Check sheet for the drawn part. Datum: minimum x, y, z corner. Units: mm. A direction names the side the tool comes from. Give positions to 0.01 mm unless a question says otherwise; leave off trailing zeros. Write each loop counter-clockwise with the first axis right and the second up, starting at its lowest first coordinate (ties: lowest second). Pieces come first, ordered by that corner, then holes. Notation, with made-up numbers: (17.5, -9) -> (36.5, -9) arc R32 cw to (36.5, 25) -> close; hole circle Ø9 at (-39.75, 36). An arc over 180 degrees is marked (long way). Answer as CSV lines item,"result". Start each with the question number.
1) Material ranges on L1, parallel to Y at x = 19, z = 31; L2, parallel to Y at x = 103.5, z = 36.5; L3, parallel to Y at x = 133.35, z = 18, recorded low to high.
2) Sectioned sample at B-B on y = 19.05. Record the cut outline in (x, z).
3) Sectioned sample at C-C on x = 133.35. Record the cut outline in (y, z) (3 decimals).
4) Sectioned sample at A-A on y = 44.5. Record the cut outline in (x, z), and give its area (3 significant figures).
5) Mould release check, pull along Z, two halves, no side actions. Record for the marked faces 4, 5, 6 and 7: released by +Z, released by -Z, zero draft, split by the parting line, or undercut.
6) Sectioned sample at D-D on z = 92. Record the cut outline in (x, y).
7) Gauge pin test, flat ends, axial feed: pin 1 Ø12 at (x, y) = (78, 94) entering from -Z; pin 2 Ø12 at (x, y) = (132.5, 86) entering from -Z; pin 3 Ø14.5 at (x, y) = (133.35, 19.05) entering from +Z; pin 4 Ø10 at (x, y) = (19.05, 19.05) entering from -Z. Record the tip position at first contact, or that the pin passes through.
8) Tool access check on the marked faces 1, 2 and 3. Record the directions out of +Z, -Z, +X, -X, +Y, -Y that give a thin tool (end or side, any length) a straight path to the whole face; none if there is none.
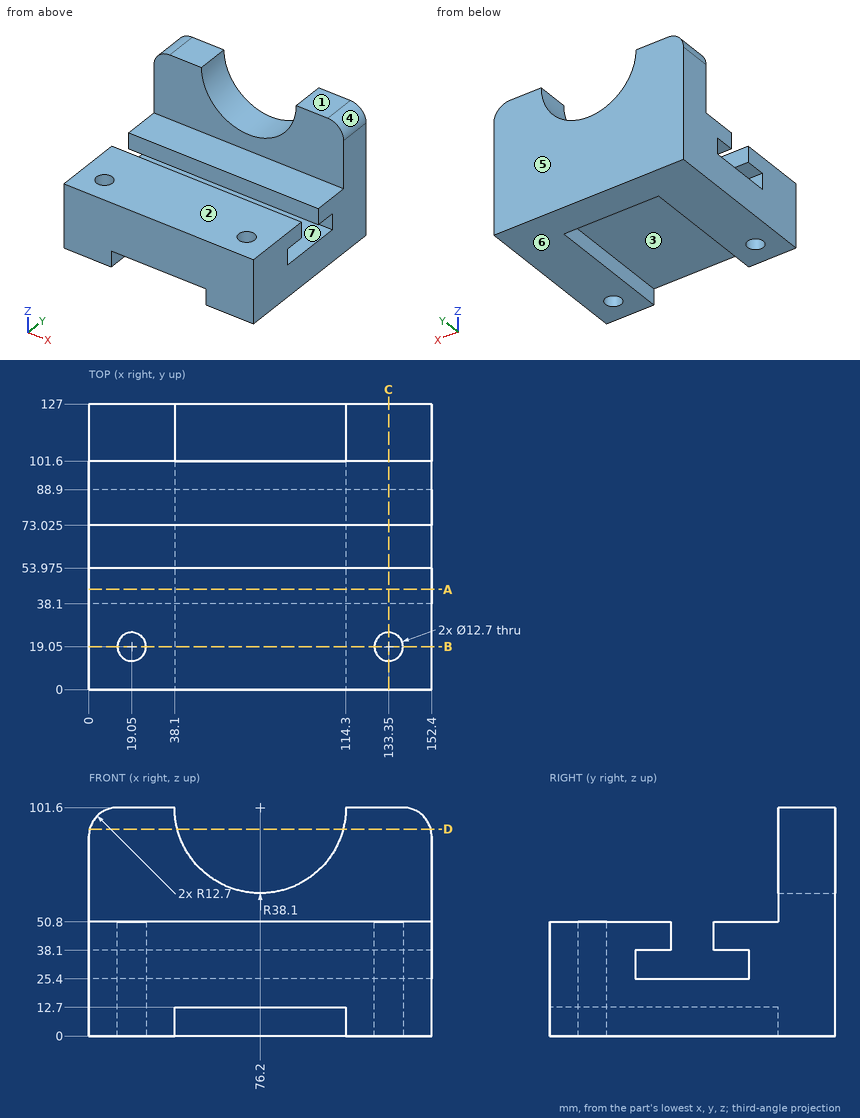
Ans:
1,L1,"y = 0 to 12.7, 25.4 to 38.1, 88.9 to 127"
1,L2,"y = 0 to 38.1, 88.9 to 127"
1,L3,"y = 0 to 12.7, 25.4 to 127"
2,outline,"(0, 0) -> (12.7, 0) -> (12.7, 50.8) -> (0, 50.8) -> close; (25.4, 0) -> (38.1, 0) -> (38.1, 12.7) -> (114.3, 12.7) -> (114.3, 0) -> (127, 0) -> (127, 50.8) -> (25.4, 50.8) -> close; (139.7, 0) -> (152.4, 0) -> (152.4, 50.8) -> (139.7, 50.8) -> close"
3,outline,"(0, 0) -> (12.7, 0) -> (12.7, 50.8) -> (0, 50.8) -> close; (25.4, 0) -> (127, 0) -> (127, 101.6) -> (101.6, 101.6) -> (101.6, 50.8) -> (73.025, 50.8) -> (73.025, 38.1) -> (88.9, 38.1) -> (88.9, 25.4) -> (38.1, 25.4) -> (38.1, 38.1) -> (53.975, 38.1) -> (53.975, 50.8) -> (25.4, 50.8) -> close"
4,outline,"(0, 0) -> (38.1, 0) -> (38.1, 12.7) -> (114.3, 12.7) -> (114.3, 0) -> (152.4, 0) -> (152.4, 25.4) -> (0, 25.4) -> close; (0, 38.1) -> (152.4, 38.1) -> (152.4, 50.8) -> (0, 50.8) -> close"
4,area,"4,840 mm²"
5,face 4,"released by +Z"
5,face 5,"zero draft"
5,face 6,"released by -Z"
5,face 7,"undercut"
6,outline,"(0.38, 101.6) -> (39.33, 101.6) -> (39.33, 127) -> (0.38, 127) -> close; (113.07, 101.6) -> (152.02, 101.6) -> (152.02, 127) -> (113.07, 127) -> close"
7,pin 1,"stops at z = 12.7"
7,pin 2,"stops at z = 0"
7,pin 3,"stops at z = 50.8"
7,pin 4,"passes through"
8,face 1,"+Z, +X, -X, +Y, -Y"
8,face 2,"+Z, +X, -X, -Y"
8,face 3,"-Z, -Y"
